from build123d import *

# Parameters (mm, degrees)
SKETCH_2_R      = 13.25
SKETCH_2_R_2    = 2.1
SKETCH_2_R_3    = 2.6
EXTRUDE_1_DEPTH = 3
FILLET_3_R      = 5


with BuildPart() as part:
    # ｽｹｯﾁ2 → ﾎﾞｽ - 押し出し1 (new body)
    with BuildSketch(Plane.XY):
        with BuildLine():
            Line((-75, 130), (-75, -10))
            Line((-75, -10), (-55, -10))
            Line((-55, -10), (-5.225491892, -21.884794596))
            ThreePointArc((-5.225491892, -21.884794596), (18.280450485, -13.117741043), (19.059394587, 11.957820787))
            Line((19.059394587, 11.957820787), (-55, 130))
            Line((-55, 130), (-75, 130))
        make_face()
        Circle(SKETCH_2_R, mode=Mode.SUBTRACT)
        with Locations((0, 17.5)):
            Circle(SKETCH_2_R_2, mode=Mode.SUBTRACT)
        with Locations((17.5, 0)):
            Circle(SKETCH_2_R_2, mode=Mode.SUBTRACT)
        with Locations((0, -17.5)):
            Circle(SKETCH_2_R_2, mode=Mode.SUBTRACT)
        with Locations((-17.5, 0)):
            Circle(SKETCH_2_R_2, mode=Mode.SUBTRACT)
        with Locations((-65, 60)):
            Circle(SKETCH_2_R_3, mode=Mode.SUBTRACT)
        with Locations((-65, 120)):
            Circle(SKETCH_2_R_3, mode=Mode.SUBTRACT)
        with Locations((-65, 0)):
            Circle(SKETCH_2_R_3, mode=Mode.SUBTRACT)
    extrude(amount=EXTRUDE_1_DEPTH)

    # ﾌｨﾚｯﾄ3
    fillet_3_edges = [part.edges().sort_by_distance(p)[0] for p in [
        (-55, 130, 1.5),
        (-55, -10, 1.5),
        (-75, -10, 1.5),
        (-75, 130, 1.5),
    ]]
    fillet(fillet_3_edges, radius=FILLET_3_R)


solid = part.part
The listing builds one solid part. Answer for the finished solid, in the listing's coordinates (mm). A direction names the side the tool comes from. Coordinates: 2 decimals unless noted, no trailing zeros. Loops run counter-clockwise (first coordinate to the right, second up) from the corner with the lowest first, then second, coordinate; pieces in that order, holes last. Notation, with made-up numbers: (12.25, 85.5) -> (50.25, 85.5) arc R25 cw to (50.25, 107.5) -> close; hole circle Ø9 at (-19.5, 29). An arc over 180 degrees is marked (long way). Write item = value, one per line. Start each with the question number.
1) A tool of negligible diameter and unlimited length cuts with its end or side. For faces 1 (the face through (-55.377, 129.392, 1.521)), 2 (the face through (-63, -10, 1)), from which of +Z, -Z, +X, -X, +Y, -Y can it reach the whole face along a straight path? Write none if from no direction.
2) A cutting plane is placed at B-B (z = 0.7). Count the separate pieces of the cut face and the enclosed holes in it, then the cut area to 3 significant figures.
3) A cutting plane is placed at D-D (y = -17.5). Give the vertices of the cut face in (x, z), then the cut area to 3 significant figures.
4) The mould has two halves that part along Y. Classify faces 3 (the face through (-64, 130, 1)), 4 (the face through (-67.6, 60.1, 1.5)), 5 (the face through (-0.273, -15.418, 1.479)), 6 (the face through (-38, 38, 3)): released by +Y, released by -Y, zero draft, split by the parting line, or undercut.
5) Straight lines are drawn through the part: line 1 (Y direction, x = -65, z = 1.5); line 2 (Y direction, x = 0, z = 1.5); line 3 (Y direction, x = -17.5, z = 1.65). For each, find the intervals that lie inside material, in ascending order. Write a range as from..to.
6) A cutting plane is placed at A-A (y = 0). Give the vertices of the cut face in (x, z).
7) Given pin 1 Ø10 at (x, y) = (-56.5, 23.5) entering from -Z; pin 2 Ø1 at (x, z) = (-33, 1.5) entering from +Y, each flat-ended and moving along its own axis, determine where each tip first touches the part or whether it passes through.
8) A cutting plane is placed at C-C (x = 4.5). Give the vertices of the cut face in (y, z), then the cut area to 3 significant figures.
Responses:
q1.face_1 = +Z, -Z, +X, +Y
q1.face_2 = +Z, -Z, -X, -Y
q2.separate_pieces = 1
q2.enclosed_holes = 8
q2.area = 8,710 mm²
q3.outline = (-23.59, 0) -> (-2.1, 0) -> (-2.1, 3) -> (-23.59, 3) -> close; (2.1, 0) -> (14.14, 0) -> (14.14, 3) -> (2.1, 3) -> close
q3.area = 101 mm²
q4.face_3 = released by +Y
q4.face_4 = undercut
q4.face_5 = undercut
q4.face_6 = zero draft
q5.line_1 = -10..-2.6, 2.6..57.4, 62.6..117.4, 122.6..130
q5.line_2 = -22.5..-19.6, -15.4..-13.25, 13.25..15.4, 19.6..42.34
q5.line_3 = -18.95..-2.1, 2.1..70.23
q6.outline = (-75, 0) -> (-67.6, 0) -> (-67.6, 3) -> (-75, 3) -> close; (-62.4, 0) -> (-19.6, 0) -> (-19.6, 3) -> (-62.4, 3) -> close; (-15.4, 0) -> (-13.25, 0) -> (-13.25, 3) -> (-15.4, 3) -> close; (13.25, 0) -> (15.4, 0) -> (15.4, 3) -> (13.25, 3) -> close; (19.6, 0) -> (22.5, 0) -> (22.5, 3) -> (19.6, 3) -> close
q7.pin_1 = 0
q7.pin_2 = 95.73
q8.outline = (-22.05, 0) -> (-12.46, 0) -> (-12.46, 3) -> (-22.05, 3) -> close; (12.46, 0) -> (35.16, 0) -> (35.16, 3) -> (12.46, 3) -> close
q8.area = 96.9 mm²
